Check sheet for the modelled part. Datum: model origin and axes. Units: mm. Face numbers are marked on the shaded views. A direction names the side the tool comes from. Round coordinates to 2 decimals unless told otherwise and drop trailing zeros. Order: outer loops, then holes, each group sorted by start corner. A loop starts at its lowest first (then second) coordinate and runs counter-clockwise, first axis right, second up. Notation, with made-up numbers: M 82.25,87.5 L 109.25,87.5 A22 cw 109.25,97.5 Z; hole C -24.5,61.25 d2. An arc over 180 degrees is marked long. One line per item, written item: value. Start each with the question number.
(1) Cross-section at B-B, the plane z = 39.5. Enter the section's corners in (x, y).
(2) Depth check by flat-ended pin: pin 1 Ø10 at (x, z) = (44.5, 40) entering from -Y; pin 2 Ø5 at (y, z) = (-1, 26) entering from +X. Enter the tip coordinate at first touch or a pass-through.
(3) Cross-section at A-A, the plane x = 32. Enter the section's corners in (y, z), and give its area (3 significant figures).
(4) Release check for a two-part mould opening along Y. For the marked faces 1, 2 and 3 record: released by +Y, released by -Y, zero draft, split by the parting line, or undercut.
(5) Thickness scan on L1, parallel to Y at x = 31, z = 5; L2, parallel to X at y = 0.5, z = 20.5; L3, parallel to Y at x = 37.5, z = 29. Record the ranges inside material, lowest first.
(6) Cross-section at D-D, the plane x = 56. Enter the section's corners in (y, z).
(7) Access from +Z, -Z, +X, -X, +Y, -Y to the whole of each face (thin tool, end or side, straight path). Record for the marked faces 4 and 5.
(8) Cross-section at C-C, the plane y = 16.5. Enter the section's corners in (x, z).
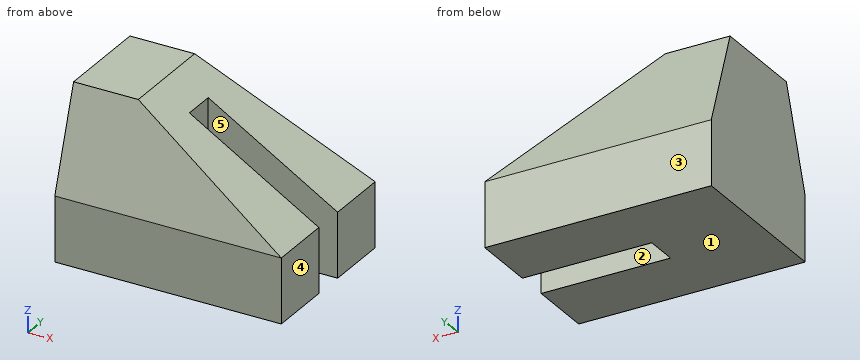
from build123d import *

# Parameters (mm, degrees)
F0_W     = 70
F0_H     = 50
F1_DEPTH = 20
F3_DEPTH = 50
F5_DEPTH = 70.001
F6_W     = 40
F6_H     = 10
F7_DEPTH = 50.001


# Not quite as in the source:
# - a pattern or mirror of a feature is missing from the dataset's text; its kind, count and spacing are read off the source's solid


with BuildPart() as f1:
    # F0 (on Top) → F1 (new body)
    with BuildSketch(Plane.XY):
        with Locations((35, 0)):
            Rectangle(F0_W, F0_H)
    extrude(amount=F1_DEPTH)

    # F2 (on face) → F3 (join, through all)
    with BuildSketch(Plane.XZ.offset(25)):
        Polygon((0, 50), (0, 20), (70, 20), (20, 50), align=None)
    extrude(amount=-F3_DEPTH)

    # F4 (on face) → F5 (cut, through all)
    with BuildSketch(Plane(origin=(0, 0, 0), x_dir=(0, -1, 0), z_dir=(-1, 0, 0))):
        Polygon((25, 20), (25, 50), (15, 50), align=None)
    f5 = extrude(amount=-F5_DEPTH, mode=Mode.SUBTRACT)

    # F5_copies: F5 across plane
    add(f5.mirror(Plane.ZX), mode=Mode.SUBTRACT)

    # F6 (on face) → F7 (cut, through all)
    with BuildSketch(Plane.XY.offset(50)):
        with Locations((50, 0)):
            Rectangle(F6_W, F6_H)
    extrude(amount=-F7_DEPTH, mode=Mode.SUBTRACT)


solid = f1.part
Values found:
1. outline: M 0,-18.5 L 37.5,-18.5 L 37.5,-5 L 30,-5 L 30,5 L 37.5,5 L 37.5,18.5 L 0,18.5 Z
2. pin 1: y = -20
2. pin 2: x = 30
3. outline: M -25,0 L -5,0 L -5,42.8 L -17.4,42.8 L -25,20 Z; M 5,0 L 25,0 L 25,20 L 17.4,42.8 L 5,42.8 Z
3. area: 1,540 mm^2
4. face 1: zero draft
4. face 2: undercut
4. face 3: released by +Y
5. L1: -25 to -5, 5 to 25
5. L2: 0 to 30
5. L3: -22 to -5, 5 to 22
6. outline: M -25,0 L -5,0 L -5,28.4 L -22.2,28.4 L -25,20 Z; M 5,0 L 25,0 L 25,20 L 22.2,28.4 L 5,28.4 Z
7. face 4: +Z, -Z, +X, +Y, -Y
7. face 5: +Z, -Z, +X
8. outline: M 0,0 L 70,0 L 70,20 L 27.5,45.5 L 0,45.5 Z
